Work out the finished part from the listing and answer in its coordinate system (mm). Face numbers are marked on the shaded views. A direction names the side the tool comes from. Round coordinates to 2 decimals unless told otherwise and drop trailing zeros. Write each loop counter-clockwise with the first axis right and the second up, starting at its lowest first coordinate (ties: lowest second). Pieces come first, ordered by that corner, then holes. Notation, with made-up numbers: M 1,88.25 L 43,88.25 A22 cw 43,108.25 Z; hole C 70.25,25 d5. An arc over 180 degrees is marked long. Answer in a Markdown table with one row per item.
```python
from build123d import *

# Parameters (mm, degrees)
SKETCH_W  = 64
SKETCH_H  = 20
PAD_DEPTH = 20


with BuildPart() as part:
    # Sketch → Pad (new body)
    with BuildSketch(Plane.XZ):
        with Locations((0, 8)):
            Rectangle(SKETCH_W, SKETCH_H)
        Polygon((-18.25, 16), (18.25, 16), (30, 7), (30, 0), (-30, 0), (-30, 7), align=None, mode=Mode.SUBTRACT)
    extrude(amount=PAD_DEPTH)


solid = part.part
```
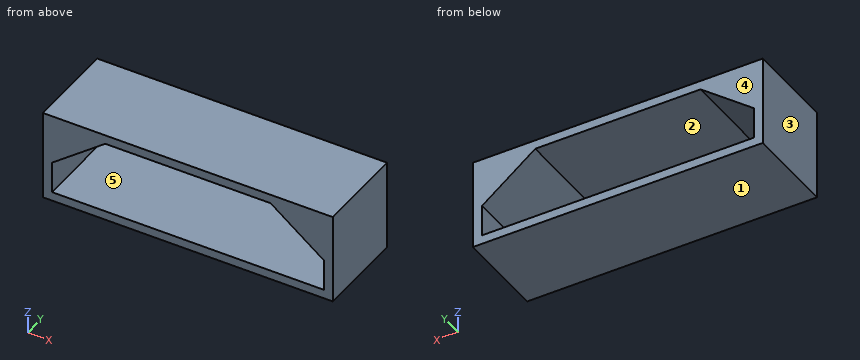
1. The part is cut by section A-A (x = -11). Determine the outline of the cut face in (y, z), plus the area to 3 significant figures.
Calculated:
| item | result |
|---|---|
| outline | M -20,-2 L 0,-2 L 0,0 L -20,0 Z; M -20,16 L 0,16 L 0,18 L -20,18 Z |
| area | 80.0 mm² |
2. Determine the mould class of the marked faces 1, 2 and 3 for opening direction Z: released by +Z, released by -Z, zero draft, split by the parting line, or undercut.
Calculated:
| item | result |
|---|---|
| face 1 | released by -Z |
| face 2 | undercut |
| face 3 | zero draft |
3. A tool of negligible diameter and unlimited length cuts with its end or side. For the marked faces 4 and 5, from which of +Z, -Z, +X, -X, +Y, -Y can it reach the whole face along a straight path? Write none if from no direction.
Calculated:
| item | result |
|---|---|
| face 4 | +Z, -Z, +X, -X, +Y |
| face 5 | +Y, -Y |
4. Consider line 1 along Z through (x, y) = (12, -1.25); line 2 along X through (y, z) = (-6.75, 2.5); line 3 along X through (y, z) = (-4, 10). Determine where each line is inside the solid, lowest interval first. Write a range as from..to.
Calculated:
| item | result |
|---|---|
| line 1 | z = -2..0, 16..18 |
| line 2 | x = -32..-30, 30..32 |
| line 3 | x = -32..-26.08, 26.08..32 |
5. The part is cut by section B-B (y = -14.5). Determine the outline of the cut face in (x, z).
Calculated:
| item | result |
|---|---|
| outline | M -32,-2 L 32,-2 L 32,18 L -32,18 Z; hole M -30,0 L 30,0 L 30,7 L 18.25,16 L -18.25,16 L -30,7 Z |
6. The part is cut by section C-C (z = 1.5). Determine the outline of the cut face in (x, y), plus the area to 3 significant figures.
Calculated:
| item | result |
|---|---|
| outline | M -32,-20 L -30,-20 L -30,0 L -32,0 Z; M 30,-20 L 32,-20 L 32,0 L 30,0 Z |
| area | 80.0 mm² |
